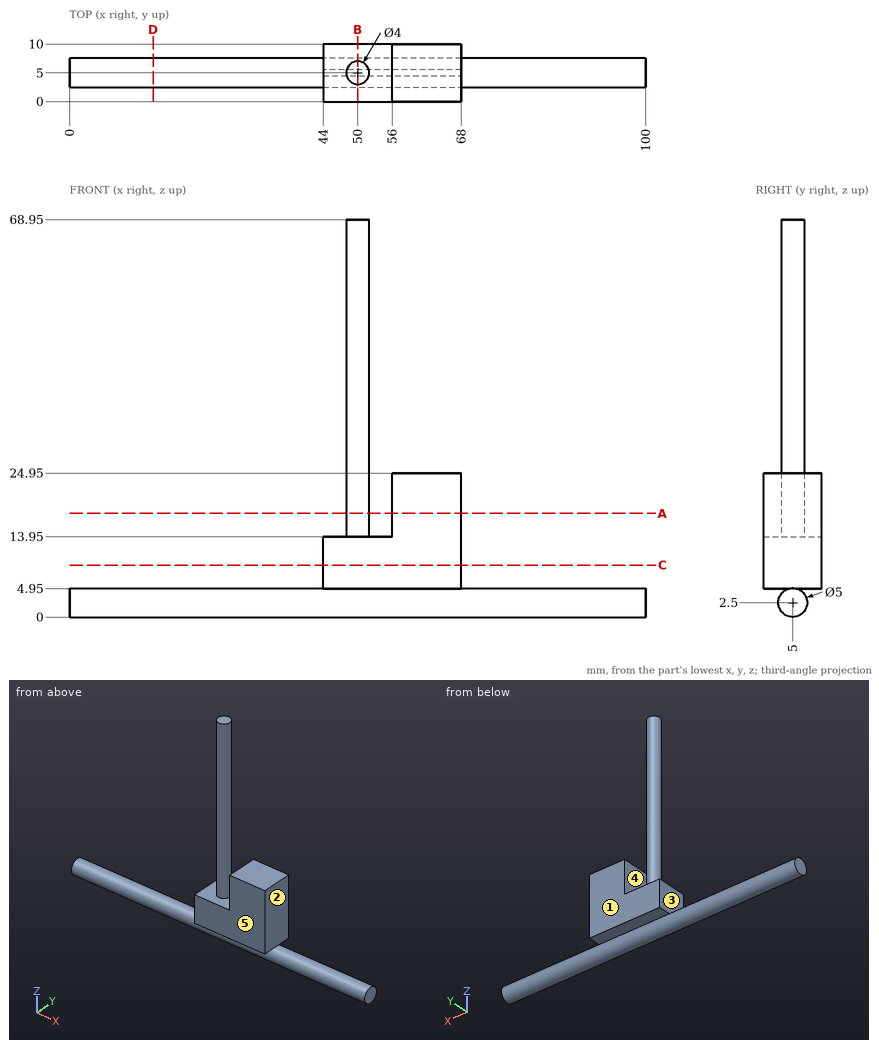
Could you check a few things on this drawing? It's one solid part, dimensions in mm from its lowest x, y, z. A direction names the side the tool comes from. Give positions to 0.01 mm unless a question says otherwise; leave off trailing zeros. Order: outer loops, then holes, each group sorted by start corner. A loop starts at its lowest first (then second) coordinate and runs counter-clockwise, first axis right, second up.
1. Suppose I cut it at A-A (z = 18). Write out the boundary of the cut face in (x, y), plus the area to 3 significant figures.
Answers below:
outline: circle Ø4 at (50, 5); (56, 0) - (68, 0) - (68, 10) - (56, 10) - close
area: 133 mm2
2. Suppose I cut it at D-D (x = 14.5). Write out the boundary of the cut face in (y, z).
Answers below:
outline: circle Ø5 at (5, 2.5)
3. For pin 1 (4 mm diameter, centred on x = 11.5, y = 6.5, fed in from +Z); pin 2 (3 mm diameter, centred on y = 7.5, z = 46.5, fed in from +X); pin 3 (1.4 mm diameter, centred on x = 53.5, y = 2.5, fed in from -Z), each with a flat end and sliding along its axis, tell me the tip position at first contact or that it passes through.
Answers below:
pin 1: stops at z = 5
pin 2: stops at x = 51.73
pin 3: stops at z = 0.77
4. Thinking about a two-plate mould opening in X: for the marked faces 3, 4 and 5, which applies, +X half, -X half, draft (parallel to the pull), parting line (faces both ways), or undercut?
Answers below:
face 3: -X half
face 4: undercut
face 5: draft
5. Suppose I cut it at C-C (z = 9). Write out the boundary of the cut face in (x, y), plus the area to 3 significant figures.
Answers below:
outline: (44, 0) - (68, 0) - (68, 10) - (44, 10) - close
area: 240 mm2
6. Suppose I cut it at B-B (x = 50). Write out the boundary of the cut face in (y, z), plus the area to 3 significant figures.
Answers below:
outline: (0, 4.95) - (4.5, 4.95) arc R2.5 ccw (long way) to (5.5, 4.95) - (10, 4.95) - (10, 13.95) - (7, 13.95) - (7, 68.95) - (3, 68.95) - (3, 13.95) - (0, 13.95) - close
area: 330 mm2
7. I need wall thicknesses on L1, parallel to Z at x = 57, y = 8.25; L2, parallel to X at y = 7, z = 5; L3, parallel to Z at x = 43, y = 4.75. Which ranges of each line are inside material? Lowest first, please.
Answers below:
L1: z = 4.95 to 24.95
L2: x = 44 to 68
L3: z = 0.01 to 4.99
8. Which directions (+Z, -Z, +X, -X, +Y, -Y) give clear straight access to the entire face, cutting with the end or side of a thin tool? Please do the marked faces 1 and 2.
Answers below:
face 1: +Z, -Z, +X, -X, +Y
face 2: +Z, +X, +Y, -Y
